Could you check a few things on this model? Use its own coordinates, in mm. A direction names the side the tool comes from. Coordinates: 2 decimals unless noted, no trailing zeros. Loops run counter-clockwise (first coordinate to the right, second up) from the corner with the lowest first, then second, coordinate; pieces in that order, holes last. Notation, with made-up numbers: (23.5, 41.5) -> (45.5, 41.5) arc R18 cw to (45.5, 51.5) -> close; hole circle Ø8 at (59, -12.5). An arc over 180 degrees is marked (long way). One line per question, with ' | ' between items. Start each with the question number.
(1) Suppose I cut it at D-D (x = -0.5). Please give me the cut outline in (y, z).
(2) If we mould it in two halves opening along Y, with no side actions, what happens to faces 5 (the face through (3.915, -1.299, 2.484)), 6 (the face through (2.1, 13.1, 4.4)), 7 (the face through (1, 10.6, 2))? For each: pulls with the +Y half, pulls with the -Y half, needs draft (parallel to the pull), parting line crosses it, or undercut.
(3) If I drill on line 1 along Y through (x, z) = (1, 4.25); line 2 along X through (y, z) = (5, 2.25); line 3 along Y through (x, z) = (2, 5.75), over which ranges is the centre line in solid material (lowest first)?
(4) Which directions (+Z, -Z, +X, -X, +Y, -Y) give clear straight access to the entire face, cutting with the end or side of a thin tool? Please do faces 1 (the face through (-2.6, 9, 2)), 2 (the face through (-2, 0, 4.9)), 3 (the face through (-1, 10, 4.9)), 4 (the face through (-0.9, 11, 2)).
(5) I'm going to push flat-ended pins straight in: pin 1 Ø1.5 at (y, z) = (6, 3.5) entering from -X; pin 2 Ø1.4 at (y, z) = (11.5, 2.5) entering from +X; pin 3 Ø1.2 at (y, z) = (7, 3) entering from +X. Where does each tip first touch, or does it pass through?
(6) Suppose I cut it at C-C (y = 2.5). Please give me the cut outline in (x, z), plus the area to 3 significant figures.
(7) Suppose I cut it at A-A (x = 1.75). Please give me the cut outline in (y, z).
(8) Suppose I cut it at B-B (z = 5.5). Please give me the cut outline in (x, y).
```python
from build123d import *

# Parameters (mm, degrees)
PAD016_DEPTH    = 4.9
SKETCH032_W     = 2.6
SKETCH032_H     = 1.2
PAD017_DEPTH    = 6.1
SKETCH031_W     = 3.5
SKETCH031_H     = 1.8
POCKET013_DEPTH = 3.4
CHAMFER_SIZE    = 1
FILLET010_R     = 1
SKETCH040_W     = 3.5
SKETCH040_H     = 1.8
POCKET016_DEPTH = 4.901


with BuildPart() as part:
    # Sketch030 → Pad016 (new body)
    with BuildSketch(Plane.XY):
        Polygon((0, 9), (0, 13.8), (2.6, 13.8), (2.6, 0), (4.2, 0), (4.2, -1.6), (1.3, -1.6), (1.3, 9), align=None)
    pad016 = extrude(amount=PAD016_DEPTH)

    # Mirrored006: Pad016 across Sketch030 V_Axis
    add(pad016.mirror(Plane(origin=(0, 0, 0), x_dir=(0, 0, 1), z_dir=(1, 0, 0))))

    # Sketch032 → Pad017 (join)
    with BuildSketch(Plane.XY):
        with Locations((2.6, 2.5)):
            Rectangle(SKETCH032_W, SKETCH032_H)
    pad017 = extrude(amount=PAD017_DEPTH)

    # Mirrored007: Pad017 across Sketch032 V_Axis
    add(pad017.mirror(Plane(origin=(0, 0, 0), x_dir=(0, 0, 1), z_dir=(1, 0, 0))))

    # Sketch031 (on Face5 of Mirrored007) → Pocket013 (cut)
    with BuildSketch(Plane.XY.offset(4.9)):
        with Locations((0.85, 11.5)):
            Rectangle(SKETCH031_W, SKETCH031_H)
    extrude(amount=-POCKET013_DEPTH, mode=Mode.SUBTRACT)

    # Chamfer
    chamfer_edges = [part.edges().sort_by_distance(p)[0] for p in [
        (-3.9, 1.9, 3.05),
        (3.9, 1.9, 3.05),
        (2.6, 6.85, 4.9),
        (2.6, 13.1, 4.9),
    ]]
    chamfer(chamfer_edges, length=CHAMFER_SIZE)

    # Fillet010
    fillet010_edges = [part.edges().sort_by_distance(p)[0] for p in [
        (4.2, -1.6, 2.45),
        (-4.2, -1.6, 2.45),
    ]]
    fillet(fillet010_edges, radius=FILLET010_R)


with BuildPart() as part_1:
    # Body004 placement: moved
    add(part.part.moved(Location((-19.5, 0, 3.95))))


with BuildPart() as part_2:
    # Clone placement: moved
    add(part_1.part.moved(Location((19.5, 0, -3.95))))

    # Sketch040 (on Face31 of Fillet010) → Pocket016 (cut, through all)
    with BuildSketch(Plane.XY.offset(4.9)):
        with Locations((0.85, 11.5)):
            Rectangle(SKETCH040_W, SKETCH040_H)
    extrude(amount=-POCKET016_DEPTH, mode=Mode.SUBTRACT)


solid = part_2.part
```
Checks:
1) outline: (9, 0) -> (10.6, 0) -> (10.6, 4.9) -> (9, 4.9) -> close; (12.4, 0) -> (13.8, 0) -> (13.8, 4.9) -> (12.4, 4.9) -> close
2) face 5: pulls with the -Y half | face 6: needs draft | face 7: undercut
3) line 1: y = 9 to 10.6, 12.4 to 13.8 | line 2: x = -2.6 to -1.3, 1.3 to 2.6 | line 3: y = 1.9 to 3.1
4) face 1: +Z, -Z, -X, +Y | face 2: +Z, +X, -X, -Y | face 3: +Z, +X, -X, +Y | face 4: +Z, -Z, +X
5) pin 1: stops at x = -2.6 | pin 2: stops at x = -0.9 | pin 3: stops at x = 2.6
6) outline: (-3.5, 0) -> (-1.3, 0) -> (-1.3, 6.1) -> (-3.5, 6.1) -> close; (1.3, 0) -> (3.5, 0) -> (3.5, 6.1) -> (1.3, 6.1) -> close | area: 26.8 mm^2
7) outline: (-1.6, 0) -> (10.6, 0) -> (10.6, 4.75) -> (3.1, 4.75) -> (3.1, 6.1) -> (1.9, 6.1) -> (1.9, 4.9) -> (-1.6, 4.9) -> close; (12.4, 0) -> (13.8, 0) -> (13.8, 4.75) -> (12.4, 4.75) -> close
8) outline: (-3.9, 2.9) -> (-2.9, 1.9) -> (-1.3, 1.9) -> (-1.3, 3.1) -> (-3.9, 3.1) -> close; (1.3, 1.9) -> (2.9, 1.9) -> (3.9, 2.9) -> (3.9, 3.1) -> (1.3, 3.1) -> close
